Autodesk Inventor part; units mm, degrees
ref_plane "YZ Plane" through (0, 0, 0) normal (1, 0, 0) x (0, 1, 0)
ref_plane "XZ Plane" through (0, 0, 0) normal (0, 1, 0) x (-1, 0, 0)
ref_plane "XY Plane" through (0, 0, 0) normal (0, 0, 1) x (1, 0, 0)
sketch "Sketch1" plane through (0, 0, 0) normal (0, 0, 1) x (1, 0, 0)
  line L0 (0, 0) -> (63.5, 0)
  line L1 (63.5, 0) -> (63.5, 19.05)
  line L2 (0, 88.9) -> (0, 0)
  circle A0 centre (6.35, 9.525) radius 2.0701
  circle A1 centre (31.75, 9.525) radius 2.0701
  circle A2 centre (57.15, 9.525) radius 2.0701
  line L3 (63.5, 19.05) -> (28.575, 88.9)
  line L4 (28.575, 88.9) -> (0, 88.9)
  line L5 (22.7162, 82.55) -> (26.3823, 76.2)
  line L6 (26.3823, 76.2) -> (22.7162, 69.85)
  line L7 (22.7162, 69.85) -> (15.3838, 69.85)
  line L8 (15.3838, 69.85) -> (11.7177, 76.2)
  line L9 (11.7177, 76.2) -> (15.3838, 82.55)
  line L10 (15.3838, 82.55) -> (22.7162, 82.55)
  point P0 (19.05, 76.2)
  dimension "d5" = 63.5
  dimension "d6" = 4.1402
  dimension "d7" = 6.35
  dimension "d8" = 9.525
  dimension "d24" = 25.4
  dimension "d29" = 88.9
  dimension "d30" = 19.05
  dimension "d31" = 28.575
  dimension "d32" = 12.7
  dimension "d34" = 19.05
  dimension "d35" = 12.7
extrude "Plate1" add sketch "Sketch1" along normal blind 3.175
sketch "Sketch3" plane through (-1.27, 88.9, -1.27) normal (-1, 0, 0) x (0, -1, 0)
  line L0 (88.9, 0) -> (0, 0)
  line L1 (0, 0) -> (0, -8.255)
  line L2 (0, -8.255) -> (88.9, -8.255)
  line L3 (88.9, -8.255) -> (88.9, 0)
edge flange "Flange2" height 12.7 angle 90 thickness 3.175 bend radius 1.27 thickness toward (-1, 0, 0) relief tear relief width 3.175 relief depth 1.5875 edges at (0, 44.45, 0) wall of the first edge with corners at (-1.27, 0, -1.27) (-1.27, 88.9, -1.27) (-1.27, 88.9, -9.525) (-1.27, 0, -9.525)
bend "Bend2"
corner "Corner2"
fillet "Fillet1" radius 3.175 5 edges at (28.575, 88.9, 1.5875) (-2.8575, 0, -9.525) (63.5, 19.05, 1.5875) (63.5, 0, 1.5875) (-2.8575, 88.9, -9.525)
equation "\"d36\" = BendReliefWidth"
equation "\"d37\" = BendReliefDepth"
equation "\"d38\" = MinimumRemnant"
equation "\"d39\" = BendRadius"
equation "\"d43\" = CornerReliefSize"
equation "\"d44\" = GapSize"
equation "\"d45\" = JacobiRadiusSize"
equation "\"BendRadius\" = Thickness"
equation "\"BendReliefWidth\" = Thickness"
equation "\"BendReliefDepth\" = 0.5 * Thickness"
equation "\"CornerReliefSize\" = 4 * Thickness"
equation "\"MinimumRemnant\" = 2 * Thickness"
equation "\"TransitionRadius\" = BendRadius"
equation "\"JacobiRadiusSize\" = BendRadius"
equation "\"GapSize\" = Thickness"
equation "\"d11\" = BendRadius"
properties part number "Spacer 3 (L-L) ipt" material "Aluminum 6061"
Check sheet for the modelled part. Datum: model origin and axes. Units: mm. A direction names the side the tool comes from. Coordinates: 2 decimals unless noted, no trailing zeros. Order: outer loops, then holes, each group sorted by start corner. A loop starts at its lowest first (then second) coordinate and runs counter-clockwise, first axis right, second up. Notation, with made-up numbers: M -34.75,12 L -29.75,12 A34 cw -29.75,48 Z; hole C -35,50 d2. An arc over 180 degrees is marked long. Write each question's results on one line, items separated by ' | '. Start each with the question number.
1. Cross-section at A-A on x = 6.35. Record the cut outline in (y, z) (3 decimals).
2. Cross-section at B-B on x = 17.5. Record the cut outline in (y, z) (3 decimals), and give its area (3 significant figures).
3. Go/stop test with flat-tipped pins: P1, Ø2.5, axis at y = 30.5, z = -5, coming from the +X side; P2, Ø3.5, axis at x = 57.15, y = 9.525, coming from the +Z side; P3, Ø1, axis at x = 22.5, y = 17.5, coming from the -Z side. Record where each tip stops, or that it passes through.
4. Material ranges on probe 1 along Y at (x, z) = (6.35, 0.95); probe 2 along Z at (x, y) = (11, 16) (3 decimals); probe 3 along X at (y, z) = (66.5, -4.5) (3 decimals), recorded low to high.
5. Cross-section at D-D on z = -2.5. Record the cut outline in (x, y) (3 decimals), and give its area (3 significant figures).
6. Access from +Z, -Z, +X, -X, +Y, -Y to the whole of each face (thin tool, end or side, straight path). Record for faces 1 (the face through (28.303, 88.413, 1.61)), 2 (the face through (24.575, 73.069, 1.565)), 3 (the face through (-1.27, 45, -5)).
7. Cross-section at C-C on y = 73.5. Record the cut outline in (x, z) (3 decimals), and give its area (3 significant figures).
Checks:
1) outline: M 0,0 L 7.455,0 L 7.455,3.175 L 0,3.175 Z; M 11.595,0 L 88.9,0 L 88.9,3.175 L 11.595,3.175 Z
2) outline: M 0,0 L 69.85,0 L 69.85,3.175 L 0,3.175 Z; M 82.55,0 L 88.9,0 L 88.9,3.175 L 82.55,3.175 Z | area: 242 mm²
3) P1: stops at x = -1.27 | P2: passes through | P3: stops at z = 0
4) probe 1: y = 0 to 7.45, 11.6 to 88.9 | probe 2: z = 0 to 3.175 | probe 3: x = -4.445 to -1.27
5) outline: M -4.445,0 L -1.27,0 L -1.27,88.9 L -4.445,88.9 Z | area: 282 mm²
6) face 1: +Z, -Z, +X, +Y | face 2: +Z, -Z | face 3: -Z, +X, +Y, -Y
7) outline: M -4.445,-9.525 L -1.27,-9.525 L -1.27,-1.27 A1.27 cw 0,0 L 13.277,0 L 13.277,3.175 L 0,3.175 A4.445 ccw -4.445,-1.27 Z; M 24.823,0 L 36.275,0 L 36.275,3.175 L 24.823,3.175 Z | area: 119 mm²
